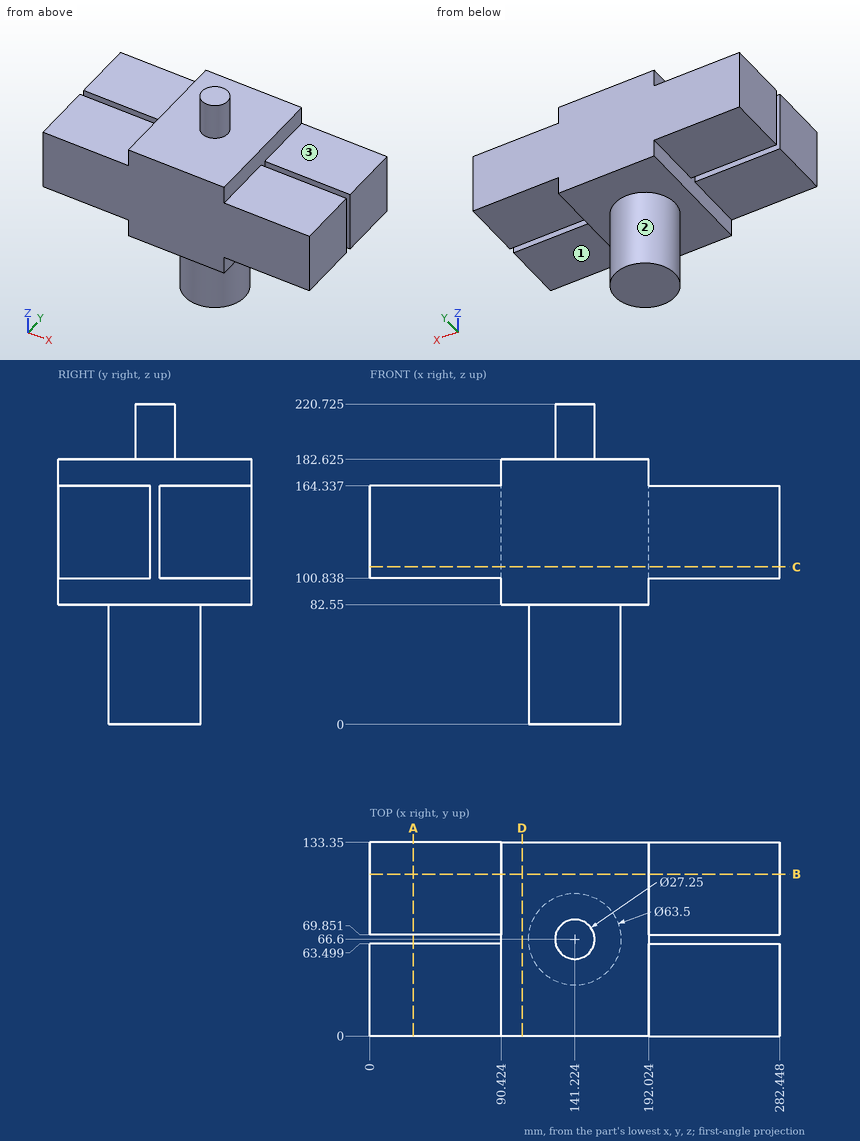
Input: dimensioned drawing with shaded views. Units: mm. Origin: part minimum x, y, z. A direction names the side the tool comes from. Give positions to 0.01 mm unless a question says otherwise; leave off trailing zeros. Loops run counter-clockwise (first coordinate to the right, second up) from the corner with the lowest first, then second, coordinate; pieces in that order, holes last. Notation, with made-up numbers: (7, 88.25) -> (63, 88.25) arc R18 ccw to (63, 97.25) -> close; hole circle Ø4 at (60.5, 44). An arc over 180 degrees is marked (long way). Use a Markdown table: item, result.
Q1. Ray query, probe 1 along Z at (x, y) = (251.5, 74.5); probe 2 along Y at (x, z) = (15.5, 114); probe 3 along X at (y, z) = (92.5, 181). Return the intervals inside material, ascending. Write a range as from..to.
Entries:
| item | result |
|---|---|
| probe 1 | z = 100.84..164.34 |
| probe 2 | y = 0..63.5, 69.85..133.35 |
| probe 3 | x = 90.42..192.02 |
Q2. Section query C-C, the plane z = 108.5. Return the cut outline in (x, y), plus the area to 3 significant figures.
Entries:
| item | result |
|---|---|
| outline | (0, 0) -> (282.45, 0) -> (282.45, 63.5) -> (192.02, 63.5) -> (192.02, 69.85) -> (282.45, 69.85) -> (282.45, 133.35) -> (0, 133.35) -> (0, 69.85) -> (90.42, 69.85) -> (90.42, 63.5) -> (0, 63.5) -> close |
| area | 36,500 mm² |
Q3. Section query D-D, the plane x = 105. Return the cut outline in (y, z) (3 decimals).
Entries:
| item | result |
|---|---|
| outline | (0, 82.55) -> (133.35, 82.55) -> (133.35, 182.625) -> (0, 182.625) -> close |
Q4. Section query A-A, the plane x = 30. Return the cut outline in (y, z), plus the area to 3 significant figures.
Entries:
| item | result |
|---|---|
| outline | (0, 100.84) -> (63.5, 100.84) -> (63.5, 164.34) -> (0, 164.34) -> close; (69.85, 100.84) -> (133.35, 100.84) -> (133.35, 164.34) -> (69.85, 164.34) -> close |
| area | 8,060 mm² |
Q5. First-contact query: P1, Ø19, axis at x = 232.5, y = 94.5, coming from the +Z side; P2, Ø4, axis at x = 127, z = 27.5, coming from the +Y side; P3, Ø2, axis at x = 171.5, z = 51, coming from the -Y side. Flat tips, straight axial feed; report the tip coordinate or a pass-through.
Entries:
| item | result |
|---|---|
| P1 | stops at z = 164.34 |
| P2 | stops at y = 95.9 |
| P3 | stops at y = 54.31 |
Q6. Access query for the marked faces 1, 2 and 3. Directions: +Z, -Z, +X, -X, +Y, -Y. A direction counts if a zero-diameter tool reaches every point of the face in a straight line with its end or side. Return the directions, or none.
Entries:
| item | result |
|---|---|
| face 1 | -Z, +X, +Y, -Y |
| face 2 | -Z |
| face 3 | +Z, +X, +Y, -Y |
Q7. Section query B-B, the plane y = 111.5. Return the cut outline in (x, z) (3 decimals).
Entries:
| item | result |
|---|---|
| outline | (0, 100.838) -> (90.424, 100.838) -> (90.424, 82.55) -> (192.024, 82.55) -> (192.024, 100.838) -> (282.448, 100.838) -> (282.448, 164.337) -> (192.024, 164.337) -> (192.024, 182.625) -> (90.424, 182.625) -> (90.424, 164.337) -> (0, 164.337) -> close |
